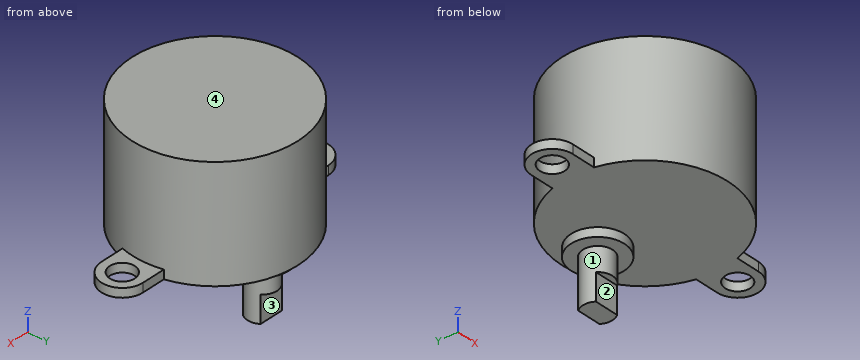
Autodesk Inventor part; units mm, degrees
ref_plane "YZ Plane" through (0, 0, 0) normal (1, 0, 0) x (0, 1, 0)
ref_plane "XZ Plane" through (0, 0, 0) normal (0, 1, 0) x (-1, 0, 0)
ref_plane "XY Plane" through (0, 0, 0) normal (0, 0, 1) x (1, 0, 0)
sketch "Sketch1" plane through (0, 0, 0) normal (0, 0, 1) x (1, 0, 0)
  circle A0 centre (0, 0) radius 14
  line L0 (0, 14) -> (0, -14)
  line L1 (-17.5, 9.3538) -> (-17.5, -9.6398)
  circle A1 centre (-17.5, 0) radius 2.1
  arc A2 (-17.5, 3.5) -> (-17.5, -3.5) centre (-17.5, 0) ccw
  line L2 (-17.5, 3.5) -> (-13.5554, 3.5)
  line L3 (-17.5, -3.5) -> (-13.5554, -3.5)
  dimension "d0" = 28
  dimension "d1" = 17.5
  dimension "d2" = 4.2
  dimension "d5" = 7
extrude "Extrusion1" add sketch "Sketch1" along normal blind 19 contours A0 L0 | L0 A0
extrude "Extrusion2" add sketch "Sketch1" along normal blind 1.5 contours A0 L3 L1 A1 L2 | L1 A1 A2
mirror "Mirror1" about plane through (0, 0, 0) normal (1, 0, 0) of "Extrusion2"
sketch "Sketch3" plane through (0, 0, 0) normal (0, 0, -1) x (-1, 0, 0)
  circle A0 centre (0, 8) radius 4.5
  circle A1 centre (0, 8) radius 2.5
  line L0 (-2, 9.5) -> (2, 9.5)
  line L1 (-2, 6.5) -> (2, 6.5)
  point P0 (0, 0)
  point P1 (0, 10.5)
  point P2 (0, 5.5)
  dimension "d8" = 9
  dimension "d9" = 8
  dimension "d10" = 5
  dimension "d12" = 1
  dimension "d13" = 1
extrude "Extrusion3" add sketch "Sketch3" along normal blind 1.5 contours A0 | A1 L1 L0 | L0 A1 | A1 L1
extrude "Extrusion4" add sketch "Sketch3" along normal blind 5.5 contours A1 L1 L0 | L0 A1 | A1 L1
extrude "Extrusion5" add sketch "Sketch3" along normal blind 10 contours A1 L1 L0
properties part number "motooor"
Work out the finished part from the listing and answer in its coordinate system (mm). Face numbers are marked on the shaded views. A direction names the side the tool comes from. Give positions to 0.01 mm unless a question says otherwise; leave off trailing zeros. Loops run counter-clockwise (first coordinate to the right, second up) from the corner with the lowest first, then second, coordinate; pieces in that order, holes last. Notation, with made-up numbers: (7.5, 5) -> (45.5, 5) arc R13 cw to (45.5, 26) -> close; hole circle Ø7 at (87, -11). An arc over 180 degrees is marked (long way). Use a Markdown table: item, result. Add a question column.
1. Flat-ended cylindrical pins translate along their axes: pin 1 Ø1.5 at (x, z) = (-7, 8.5) entering from -Y; pin 2 Ø0.5 at (x, y) = (-0.5, 6) entering from -Z; pin 3 Ø6 at (x, z) = (-6.5, 0) entering from -Y. Find the tip coordinate at first contact, or state that the pin passes through.
2. Section B-B on x = 0 is taken. Determine the outline of the cut face in (y, z).
3. Find the intervals of material crossed by probe 1 along X at (y, z) = (0, 0.65); probe 2 along Y at (x, z) = (17.5, 0.35); probe 3 along Z at (x, y) = (9, -5.75), in increasing order.
4. Section A-A on y = 0 is taken. Determine the outline of the cut face in (x, z).
5. For the marked faces 1, 2, 3 and 4, determine the directions among +Z, -Z, +X, -X, +Y, -Y from which every point of the face is accessible in a straight line to the end or side of a thin tool.
6. Section C-C on x = -16 is taken. Determine the outline of the cut face in (y, z).
7. Section D-D on z = 13.5 is taken. Determine the outline of the cut face in (x, y).
Results below:
| question | item | result |
|---|---|---|
| 1 | pin 1 | stops at y = -12.53 |
| 1 | pin 2 | stops at z = -5.5 |
| 1 | pin 3 | stops at y = -13.56 |
| 2 | outline | (-14, 0) -> (3.5, 0) -> (3.5, -1.5) -> (5.5, -1.5) -> (5.5, -5.5) -> (6.5, -5.5) -> (6.5, -10) -> (9.5, -10) -> (9.5, -5.5) -> (10.5, -5.5) -> (10.5, -1.5) -> (12.5, -1.5) -> (12.5, 0) -> (14, 0) -> (14, 19) -> (-14, 19) -> close |
| 3 | probe 1 | x = -21 to -19.6, -15.4 to 15.4, 19.6 to 21 |
| 3 | probe 2 | y = -3.5 to -2.1, 2.1 to 3.5 |
| 3 | probe 3 | z = 0 to 19 |
| 4 | outline | (-21, 0) -> (-19.6, 0) -> (-19.6, 1.5) -> (-21, 1.5) -> close; (-15.4, 0) -> (15.4, 0) -> (15.4, 1.5) -> (14, 1.5) -> (14, 19) -> (-14, 19) -> (-14, 1.5) -> (-15.4, 1.5) -> close; (19.6, 0) -> (21, 0) -> (21, 1.5) -> (19.6, 1.5) -> close |
| 5 | face 1 | -Z |
| 5 | face 2 | -Z, +X, -X, -Y |
| 5 | face 3 | -Z, +X, -X, +Y |
| 5 | face 4 | +Z, +X, -X, +Y, -Y |
| 6 | outline | (-3.5, 0) -> (-1.47, 0) -> (-1.47, 1.5) -> (-3.5, 1.5) -> close; (1.47, 0) -> (3.5, 0) -> (3.5, 1.5) -> (1.47, 1.5) -> close |
| 7 | outline | circle Ø28 at (0, 0) |
